The drawing under review shows one solid part. Ordinate dimensions are in mm from its lowest x, y, z. A direction names the side the tool comes from. Round coordinates to 2 decimals unless told otherwise and drop trailing zeros. Order: outer loops, then holes, each group sorted by start corner. A loop starts at its lowest first (then second) coordinate and runs counter-clockwise, first axis right, second up. Notation, with made-up numbers: (24.25, 84.5) - (80.25, 84.5) arc R22 cw to (80.25, 101.5) - close; hole circle Ø8 at (45.5, 10.25). An arc over 180 degrees is marked (long way). One line per question, with ' | ' between items.
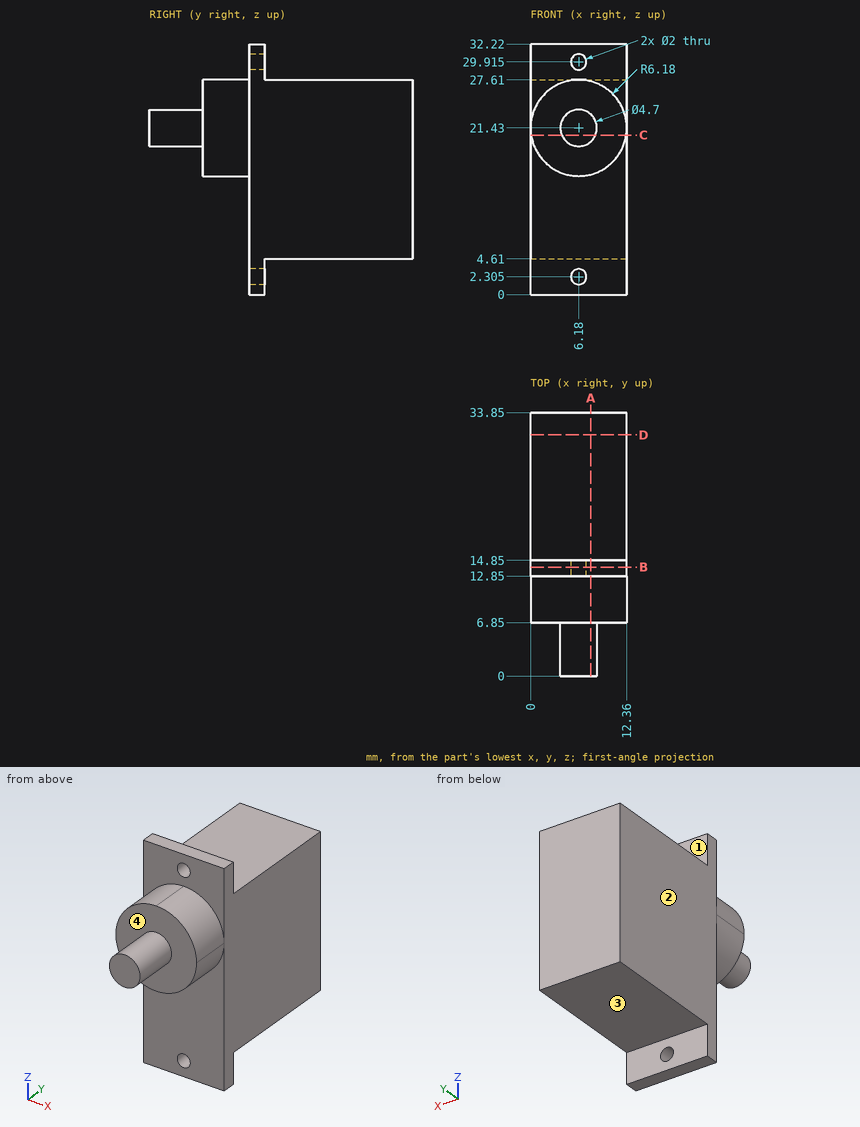
(1) We need section C-C on z = 20.5. State the section outline as (x, y) points.
Output values:
outline: (0, 12.85) - (0.07, 12.85) - (0.07, 6.85) - (4.02, 6.85) - (4.02, 0) - (8.34, 0) - (8.34, 6.85) - (12.29, 6.85) - (12.29, 12.85) - (12.36, 12.85) - (12.36, 33.85) - (0, 33.85) - close
(2) For probe 1 along Z at (x, y) = (6.18, 13.9) (3 decimals); probe 2 along Z at (x, y) = (1, 31); probe 3 along Y at (x, z) = (7.25, 27), list the stretches that pass through material, from the lowest coordinate up. Write a range as [from, to].
Output values:
probe 1: [0, 1.305], [3.305, 28.915], [30.915, 32.22] | probe 2: [4.61, 27.61] | probe 3: [6.85, 33.85]
(3) For the marked faces 1, 2, 3 and 4, list the 3-axis set-ups (+Z, -Z, +X, -X, +Y, -Y) from which the entire face can be reached by the end or side of a thin tool; tool diameter is ignored.
Output values:
face 1: +Z, +X, -X, +Y | face 2: +Z, -Z, -X, +Y, -Y | face 3: -Z, +X, -X, +Y | face 4: -Y
(4) We need section B-B on y = 14. State the section outline as (x, z) points (3 decimals).
Output values:
outline: (0, 0) - (12.36, 0) - (12.36, 32.22) - (0, 32.22) - close; hole circle Ø2 at (6.18, 2.305); hole circle Ø2 at (6.18, 29.915)
(5) We need section A-A on x = 7.75. State the section outline as (y, z) points.
Output values:
outline: (0, 19.68) - (6.85, 19.68) - (6.85, 15.45) - (12.85, 15.45) - (12.85, 0) - (14.85, 0) - (14.85, 4.61) - (33.85, 4.61) - (33.85, 27.61) - (14.85, 27.61) - (14.85, 32.22) - (12.85, 32.22) - (12.85, 27.41) - (6.85, 27.41) - (6.85, 23.18) - (0, 23.18) - close
(6) Insertion check: pin 1 (6 mm diameter, centred on x = 5.5, y = 23, fed in from +Z); pin 2 (4 mm diameter, centred on x = 4, y = 19.5, fed in from -Z); pin 3 (5 mm diameter, centred on x = 8.5, z = 30.5, fed in from +Y). Each pin has a flat end and moves straight along its axis. Give the tip position at first contact, or say it passes through.
Output values:
pin 1: z = 27.61 | pin 2: z = 4.61 | pin 3: y = 14.85
(7) We need section D-D on y = 31. State the section outline as (x, z) points, plus the area to 3 significant figures.
Output values:
outline: (0, 4.61) - (12.36, 4.61) - (12.36, 27.61) - (0, 27.61) - close | area: 284 mm^2
